```python
from build123d import *

# Parameters (mm, degrees)
F0_R     = 1.25
F0_W     = 10.5
F0_H     = 3.5
F0_R_2   = 3
F0_R_3   = 1.75
F1_DEPTH = 5
F2_DEPTH = 2
F3_DEPTH = 2.5


with BuildPart() as f1:
    # F0 (on Top) → F1 (new body)
    with BuildSketch(Plane.XY):
        with BuildLine():
            Line((29.3314352036, 17.5223795399), (-29.6685647964, 17.5223795399))
            ThreePointArc((-29.6685647964, 17.5223795399), (-33.9112054836, 15.765020227), (-35.6685647964, 11.5223795399))
            Line((-35.6685647964, 11.5223795399), (-35.6685647964, -12.4776204601))
            ThreePointArc((-35.6685647964, -12.4776204601), (-33.9112054836, -16.7202611472), (-29.6685647964, -18.4776204601))
            Line((-29.6685647964, -18.4776204601), (29.3314352036, -18.4776204601))
            ThreePointArc((29.3314352036, -18.4776204601), (33.5740758907, -16.7202611472), (35.3314352036, -12.4776204601))
            Line((35.3314352036, -12.4776204601), (35.3314352036, 11.5223795399))
            ThreePointArc((35.3314352036, 11.5223795399), (33.5740758907, 15.765020227), (29.3314352036, 17.5223795399))
        make_face()
        with Locations((-27.4148993194, -7.3692747392)):
            Circle(F0_R, mode=Mode.SUBTRACT)
        with Locations((-12.4803110957, -9.3660038244)):
            Rectangle(F0_W, F0_H, mode=Mode.SUBTRACT)
        with Locations((1.526786318, -9.4208057884)):
            Rectangle(F0_W, F0_H, mode=Mode.SUBTRACT)
        with BuildLine():
            Line((12.8467483446, -8.7025752291), (12.8467483446, -7.2025752291))
            Line((12.8467483446, -7.2025752291), (16.6563325848, -7.2025752291))
            ThreePointArc((16.6563325848, -7.2025752291), (21.3467483446, -3.2025752291), (26.0371641044, -7.2025752291))
            Line((26.0371641044, -7.2025752291), (29.8467483446, -7.2025752291))
            Line((29.8467483446, -7.2025752291), (29.8467483446, -8.7025752291))
            Line((29.8467483446, -8.7025752291), (26.0371641044, -8.7025752291))
            ThreePointArc((26.0371641044, -8.7025752291), (21.3467483446, -12.7025752291), (16.6563325848, -8.7025752291))
            Line((16.6563325848, -8.7025752291), (12.8467483446, -8.7025752291))
        make_face(mode=Mode.SUBTRACT)
        with Locations((-28.6685647964, 10.5223795399)):
            Circle(F0_R_2, mode=Mode.SUBTRACT)
        with BuildLine():
            ThreePointArc((30.3314352036, 10.5223795399), (27.3314352036, 7.5223795399), (24.3314352036, 10.5223795399))
            ThreePointArc((24.3314352036, 10.5223795399), (27.3314352036, 13.5223795399), (30.3314352036, 10.5223795399))
        make_face(mode=Mode.SUBTRACT)
        with Locations((-28.6685647964, 10.5223795399)):
            Circle(F0_R_2)
        with Locations((-28.6685647964, 10.5223795399)):
            Circle(F0_R_3, mode=Mode.SUBTRACT)
        with BuildLine():
            Line((26.0371641044, -8.7025752291), (16.6563325848, -8.7025752291))
            ThreePointArc((16.6563325848, -8.7025752291), (21.3467483446, -12.7025752291), (26.0371641044, -8.7025752291))
        make_face()
        with BuildLine():
            ThreePointArc((26.0371641044, -7.2025752291), (21.3467483446, -3.2025752291), (16.6563325848, -7.2025752291))
            Line((16.6563325848, -7.2025752291), (26.0371641044, -7.2025752291))
        make_face()
        with BuildLine():
            ThreePointArc((30.3314352036, 10.5223795399), (27.3314352036, 13.5223795399), (24.3314352036, 10.5223795399))
            ThreePointArc((24.3314352036, 10.5223795399), (27.3314352036, 7.5223795399), (30.3314352036, 10.5223795399))
        make_face()
        with BuildLine():
            ThreePointArc((25.5814352036, 10.5223795399), (27.3314352036, 12.2723795399), (29.0814352036, 10.5223795399))
            ThreePointArc((29.0814352036, 10.5223795399), (27.3314352036, 8.7723795399), (25.5814352036, 10.5223795399))
        make_face(mode=Mode.SUBTRACT)
    extrude(amount=-F1_DEPTH)

    # F0 (on Top) → F2 (cut)
    with BuildSketch(Plane.XY):
        with Locations((-28.6685647964, 10.5223795399)):
            Circle(F0_R_2)
        with Locations((-28.6685647964, 10.5223795399)):
            Circle(F0_R_3, mode=Mode.SUBTRACT)
        with BuildLine():
            ThreePointArc((30.3314352036, 10.5223795399), (27.3314352036, 13.5223795399), (24.3314352036, 10.5223795399))
            ThreePointArc((24.3314352036, 10.5223795399), (27.3314352036, 7.5223795399), (30.3314352036, 10.5223795399))
        make_face()
        with BuildLine():
            ThreePointArc((25.5814352036, 10.5223795399), (27.3314352036, 12.2723795399), (29.0814352036, 10.5223795399))
            ThreePointArc((29.0814352036, 10.5223795399), (27.3314352036, 8.7723795399), (25.5814352036, 10.5223795399))
        make_face(mode=Mode.SUBTRACT)
    extrude(amount=-F2_DEPTH, mode=Mode.SUBTRACT)

    # F0 (on Top) → F3 (cut)
    with BuildSketch(Plane.XY):
        with BuildLine():
            Line((26.0371641044, -8.7025752291), (16.6563325848, -8.7025752291))
            ThreePointArc((16.6563325848, -8.7025752291), (21.3467483446, -12.7025752291), (26.0371641044, -8.7025752291))
        make_face()
        with BuildLine():
            ThreePointArc((26.0371641044, -7.2025752291), (21.3467483446, -3.2025752291), (16.6563325848, -7.2025752291))
            Line((16.6563325848, -7.2025752291), (26.0371641044, -7.2025752291))
        make_face()
    extrude(amount=-F3_DEPTH, mode=Mode.SUBTRACT)


solid = f1.part
```
Source: CAD feature listing. Evaluate the final solid. Frame: model axes, mm. A direction names the side the tool comes from. Give positions to 0.01 mm unless a question says otherwise; leave off trailing zeros. Write each loop counter-clockwise with the first axis right and the second up, starting at its lowest first coordinate (ties: lowest second). Pieces come first, ordered by that corner, then holes.
1. Section query D-D (x = -10). Return the cut outline in (y, z), then the cut area to 4 significant figures.
2. Pull-direction query (X, two-part tool) for faces 1 (the face through (33.62, 15.72, -2.46)), 2 (the face through (-17.73, -9, -2)), 3 (the face through (-1, -18.478, -2)); classes: +X half, -X half, draft (parallel to the pull), parting line (faces both ways), or undercut.
3. Section query B-B (z = -0.85). Return the cut outline in (x, y).
4. First-contact query: pin 1 (5.5 mm diameter, centred on x = -28.67, y = 10.52, fed in from +Z); pin 2 (1.2 mm diameter, centred on x = 21, y = -4.5, fed in from +Z). Flat tips, straight axial feed; report the tip coordinate or a pass-through.
5. Section query A-A (x = 15). Return the cut outline in (y, z).
6. Material intervals for line 1 along Y through (x, z) = (-8, -0.55); line 2 along Y through (x, z) = (3, -1.95); line 3 along X through (y, z) = (10.5, -3.8), sorted ascending.
7. Access query for faces 4 (the face through (29.847, -8, -2)), 5 (the face through (-31.666, 10.654, -0.986)), 6 (the face through (-1, 0, -5)). Directions: +Z, -Z, +X, -X, +Y, -Y. A direction counts if a zero-diameter tool reaches every point of the face in a straight line with its end or side. Return the directions, or none.
8. Section query C-C (x = 27). Return the cut outline in (y, z), then the cut area to 3 significant figures.
Output values:
1. outline: (-18.48, -5) - (-11.12, -5) - (-11.12, 0) - (-18.48, 0) - close; (-7.62, -5) - (17.52, -5) - (17.52, 0) - (-7.62, 0) - close
1. area: 162.5 mm2
2. face 1: +X half
2. face 2: undercut
2. face 3: draft
3. outline: (-35.67, -12.48) arc R6 ccw to (-29.67, -18.48) - (29.33, -18.48) arc R6 ccw to (35.33, -12.48) - (35.33, 11.52) arc R6 ccw to (29.33, 17.52) - (-29.67, 17.52) arc R6 ccw to (-35.67, 11.52) - close; hole circle Ø6 at (-28.67, 10.52); hole circle Ø2.5 at (-27.41, -7.37); hole (-17.73, -11.12) - (-7.23, -11.12) - (-7.23, -7.62) - (-17.73, -7.62) - close; hole (-3.72, -11.17) - (6.78, -11.17) - (6.78, -7.67) - (-3.72, -7.67) - close; hole (12.85, -8.7) - (16.66, -8.7) arc R4.75 ccw to (26.04, -8.7) - (29.85, -8.7) - (29.85, -7.2) - (26.04, -7.2) arc R4.75 ccw to (16.66, -7.2) - (12.85, -7.2) - close; hole circle Ø6 at (27.33, 10.52)
4. pin 1: stops at z = -2
4. pin 2: stops at z = -2.5
5. outline: (-18.48, -5) - (-8.7, -5) - (-8.7, 0) - (-18.48, 0) - close; (-7.2, -5) - (17.52, -5) - (17.52, 0) - (-7.2, 0) - close
6. line 1: y = -18.48 to -11.12, -7.62 to 17.52
6. line 2: y = -18.48 to -11.17, -7.67 to 17.52
6. line 3: x = -35.67 to -30.42, -26.92 to 25.58, 29.08 to 35.33
7. face 4: +Z, -Z
7. face 5: +Z
7. face 6: -Z, +X, -X, +Y, -Y
8. outline: (-18.48, -5) - (-8.7, -5) - (-8.7, 0) - (-18.48, 0) - close; (-7.2, -5) - (8.8, -5) - (8.8, -2) - (7.54, -2) - (7.54, 0) - (-7.2, 0) - close; (12.24, -5) - (17.52, -5) - (17.52, 0) - (13.5, 0) - (13.5, -2) - (12.24, -2) - close
8. area: 150 mm2
